For this review, take the finished solid that the model builds, in its own axes (mm). A direction names the side the tool comes from. Give positions to 0.01 mm unless a question says otherwise; leave off trailing zeros. Order: outer loops, then holes, each group sorted by start corner. A loop starts at its lowest first (then second) coordinate and runs counter-clockwise, first axis right, second up. Notation, with made-up numbers: (-29.75, -34.75) - (-5.75, -34.75) arc R19 cw to (-5.75, -27.75) - close; hole circle Ø4 at (61, 79). An arc over 180 degrees is marked (long way). One line per item, written item: value.
```python
from build123d import *

# Parameters (mm, degrees)
SKETCH2_R           = 2.5
BOSS_EXTRUDE1_DEPTH = 5
BOSS_EXTRUDE2_START = -8
SKETCH3_R           = 2.5
SKETCH3_R_2         = 0.5
BOSS_EXTRUDE2_DEPTH = 8
SKETCH4_R           = 2.5
SKETCH4_R_2         = 0.5
BOSS_EXTRUDE3_DEPTH = 10


with BuildPart() as part:
    # Sketch2 → Boss-Extrude1 (new body)
    with BuildSketch(Plane.XY):
        with BuildLine():
            Line((-37, 4), (0, 4))
            ThreePointArc((0, 4), (1.846994453, 3.548043333), (3.276608177, 2.294305745))
            Line((3.276608177, 2.294305745), (8.438796104, -5.078062653))
            ThreePointArc((8.438796104, -5.078062653), (8.537284882, -9.519161483), (4.473211982, -11.31258567))
            Line((4.473211982, -11.31258567), (-37.688975946, -3.940217271))
            ThreePointArc((-37.688975946, -3.940217271), (-40.985026291, 0.345782384), (-37, 4))
        make_face()
        with Locations((-37, 0)):
            Circle(SKETCH2_R, mode=Mode.SUBTRACT)
        Circle(SKETCH2_R, mode=Mode.SUBTRACT)
        with Locations((5.162187927, -7.372368399)):
            Circle(SKETCH2_R, mode=Mode.SUBTRACT)
    extrude(amount=BOSS_EXTRUDE1_DEPTH)

    # Sketch3 → Boss-Extrude2 (add)
    with BuildSketch(Plane.XY.offset(5).offset(BOSS_EXTRUDE2_START)):
        with Locations((5.162187927, -7.372368399)):
            Circle(SKETCH3_R)
        with Locations((5.162187927, -7.372368399)):
            Circle(SKETCH3_R_2, mode=Mode.SUBTRACT)
    extrude(amount=BOSS_EXTRUDE2_DEPTH)

    # Sketch4 → Boss-Extrude3 (add)
    with BuildSketch(Plane(origin=(0, 0, 0), x_dir=(-1, 0, 0), z_dir=(0, 0, -1))):
        Circle(SKETCH4_R)
        Circle(SKETCH4_R_2, mode=Mode.SUBTRACT)
    extrude(amount=-BOSS_EXTRUDE3_DEPTH)


solid = part.part
```
(1) Take a section at A-A (y = -1.25). Write out the cut boundary in (x, z).
Answers below:
outline: (-40.8, 0) - (-39.17, 0) - (-39.17, 5) - (-40.8, 5) - close; (-34.83, 0) - (5.76, 0) - (5.76, 5) - (2.17, 5) - (2.17, 10) - (-2.17, 10) - (-2.17, 5) - (-34.83, 5) - close
(2) For P1, Ø5, axis at x = -19, y = -9, coming from the -Z side; P2, Ø1.5, axis at y = -2.5, z = 1.5, coming from the -X side; P3, Ø4, axis at x = -37, y = 0, coming from the +Z side; P4, Ø1.5, axis at y = 1, z = 2, coming from the +X side, all flat-tipped, find the tip position at first contact; note any pin that passes through.
Answers below:
P1: stops at z = 0
P2: stops at x = -40.6
P3: passes through
P4: stops at x = 4.71
(3) Draft analysis for pull direction Y (two halves, no side actions). For faces 4 (the face through (5.097, -6.877, 0.944)), 5 (the face through (8.572, -9.463, 2.465)), 6 (the face through (-16, -2, 5)), state which applies: pulls with the +Y half, pulls with the -Y half, needs draft (parallel to the pull), parting line crosses it, or undercut.
Answers below:
face 4: undercut
face 5: parting line crosses it
face 6: needs draft
(4) Take a section at C-C (x = -36). Write out the cut boundary in (y, z).
Answers below:
outline: (-4.24, 0) - (-2.29, 0) - (-2.29, 5) - (-4.24, 5) - close; (2.29, 0) - (4, 0) - (4, 5) - (2.29, 5) - close
(5) Machinability: for faces 1 (the face through (0.54, -2.44, 7.46)), 2 (the face through (-16.31, -7.68, 2.46)), 3 (the face through (4.8, -4.9, -1.5)), which of the approach directions +Z, -Z, +X, -X, +Y, -Y give a long, thin tool a straight path to every point of the face, cutting with its end or side? Answer none if there is none.
Answers below:
face 1: +Z
face 2: +Z, -Z, -X, -Y
face 3: -Z
(6) Take a section at D-D (z = 6). Write out the cut boundary in (x, y).
Answers below:
outline: circle Ø5 at (0, 0); hole circle Ø1 at (0, 0)
(7) Take a section at B-B (z = 3.5). Write out the cut boundary in (x, y).
Answers below:
outline: (-37.69, -3.94) - (4.47, -11.31) arc R4 ccw to (8.44, -5.08) - (3.28, 2.29) arc R4 ccw to (0, 4) - (-37, 4) arc R4 ccw to start; hole circle Ø5 at (-37, 0); hole circle Ø1 at (0, 0); hole circle Ø1 at (5.16, -7.37)
(8) Wall thickness on line 1 (Z direction, x = -3.5, y = -3); line 2 (Z direction, x = 7.5, y = -6.75); line 3 (Y direction, x = -37, z = 1.25): over which ranges is each line inside the solid? List them lowest first. Write a range as from..to.
Answers below:
line 1: z = 0..5
line 2: z = -3..5
line 3: y = -4.06..-2.5, 2.5..4
